Can you work these out from the drawing? Everything is in mm from the part's minimum corner. A direction names the side the tool comes from. Round coordinates to 2 decimals unless told otherwise and drop trailing zeros. Loops run counter-clockwise (first coordinate to the right, second up) from the corner with the lowest first, then second, coordinate; pieces in that order, holes last. Notation, with made-up numbers: (55, 49) -> (94, 49) arc R17 cw to (94, 76) -> close; hole circle Ø4 at (-5.5, -14.75). An arc over 180 degrees is marked (long way). One line per item, written item: value.
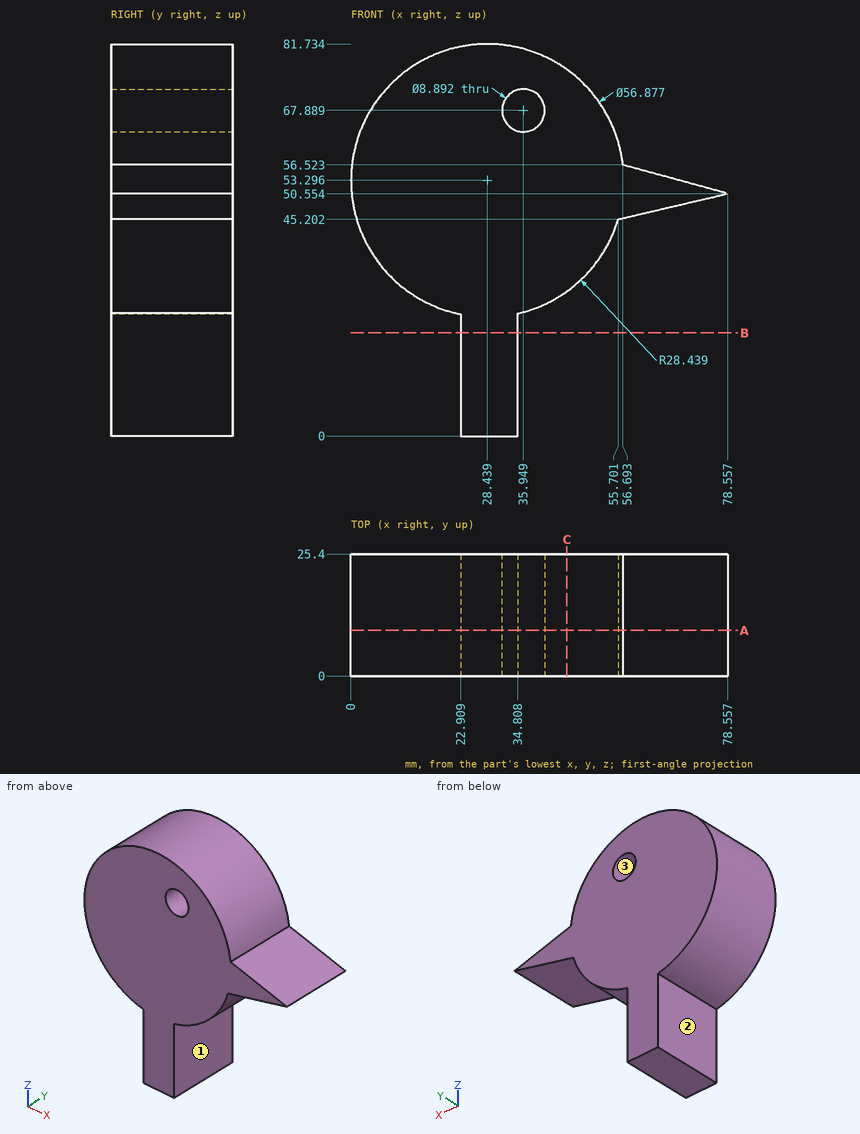
Item 1: For the marked faces 1, 2 and 3, which set-ups out of +Z, -Z, +X, -X, +Y, -Y let a thin tool reach every point of the face, with its end or its side?
Output:
face 1: -Z, +X, +Y, -Y
face 2: -Z, -X, +Y, -Y
face 3: +Y, -Y
Item 2: If we section it at A-A on y = 9.5: List the corners of the cut face in (x, z) for me (1 decimal).
Output:
outline: (22.9, 0) -> (34.8, 0) -> (34.8, 25.6) arc R28.4 ccw to (55.7, 45.2) -> (78.6, 50.6) -> (56.7, 56.5) arc R28.4 ccw (long way) to (22.9, 25.4) -> close; hole circle Ø8.9 at (35.9, 67.9)
Item 3: I need wall thicknesses on line 1 (X direction, y = 10, z = 15.5); line 2 (Z direction, x = 18.5, y = 4.5); line 3 (X direction, y = 21.25, z = 35.5) (1 decimal). Which ranges of each line are inside material? Lowest first, please. Write a range as from..to.
Output:
line 1: x = 22.91..34.81
line 2: z = 26.65..79.94
line 3: x = 6.3..50.6
Item 4: If we section it at C-C on x = 45: List the corners of the cut face in (y, z) for me (1 decimal), plus the area to 3 significant figures.
Output:
outline: (0, 30.2) -> (25.4, 30.2) -> (25.4, 76.4) -> (0, 76.4) -> close
area: 1,170 mm²
Item 5: Will these pins go through, and if not, where does the flat tip stop? pin 1 Ø5.5 at (x, z) = (35.95, 67.89) entering from -Y; pin 2 Ø10 at (y, z) = (16.5, 67.5) entering from -X; pin 3 Ø8 at (x, y) = (66.5, 19.5) entering from +Z; pin 4 Ø12 at (y, z) = (18, 36.5) entering from -X.
Output:
pin 1: passes through
pin 2: stops at x = 1.53
pin 3: stops at z = 54.94
pin 4: stops at x = 2.13
Item 6: If we section it at B-B on z = 21.5: List the corners of the cut face in (x, y) for me.
Output:
outline: (22.91, 0) -> (34.81, 0) -> (34.81, 25.4) -> (22.91, 25.4) -> close
